Design review of the part built by this model. Coordinates are the model's own, in mm. Face numbers are marked on the shaded views. A direction names the side the tool comes from. Coordinates: 2 decimals unless noted, no trailing zeros. Loops run counter-clockwise (first coordinate to the right, second up) from the corner with the lowest first, then second, coordinate; pieces in that order, holes last. Notation, with made-up numbers: M 71.25,-21 L 104.25,-21 A27 cw 104.25,5 Z; hole C 8.25,79.5 d11. An arc over 180 degrees is marked long. Write item = value, one per line. Start each with the question number.
Autodesk Inventor part; units mm, degrees
ref_plane "YZ Plane" through (0, 0, 0) normal (1, 0, 0) x (0, 1, 0)
ref_plane "XZ Plane" through (0, 0, 0) normal (0, 1, 0) x (-1, 0, 0)
ref_plane "XY Plane" through (0, 0, 0) normal (0, 0, 1) x (1, 0, 0)
sketch "Skizze1" plane through (0, 0, 0) normal (1, 0, 0) x (0, 1, 0)
  line L0 (-12.2718, -10.7427) -> (15.7282, -10.7427)
  line L1 (15.7282, -10.7427) -> (15.7282, -12.7427)
  line L2 (15.7282, -12.7427) -> (-14.2718, -12.7427)
  line L3 (-14.2718, -12.7427) -> (-14.2718, 3.7136)
  line L4 (-14.2718, -12.7427) -> (-6.9903, -12.7427)
  line L5 (-12.2718, -10.7427) -> (-12.2718, 17.2573)
  line L6 (-12.2718, 17.2573) -> (-14.2718, 17.2573)
  line L7 (-14.2718, 17.2573) -> (-14.2718, -12.7427)
  point P0 (0, 0)
  dimension "d0" = 30
  dimension "d1" = 30
  dimension "d2" = 2
  dimension "d3" = 2
extrude "Extrusion1" add sketch "Skizze1" along normal mid plane 30
properties part number "Winkel"
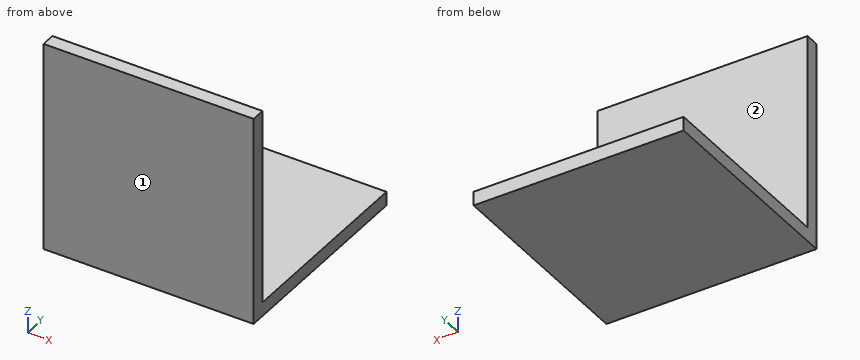
Q1. Add section B-B on x = 3. State the section outline as (y, z) points.
Q2. Add section A-A on y = 7.5. State the section outline as (x, z) points, plus the area to 3 significant figures.
Q3. To check wall thickness, follow line 1 (Y direction, x = 1, z = 8.25); line 2 (Z direction, x = -6, y = -7.5). State the ranges of each line that lie inside material, in increasing order. Write a range as from..to.
Q4. For the marked faces 1 and 2, list the 3-axis set-ups (+Z, -Z, +X, -X, +Y, -Y) from which the entire face can be reached by the end or side of a thin tool; tool diameter is ignored.
Q5. Add section C-C on z = 7. State the section outline as (x, y) points.
Q6. Clearance check with flat-ended pins moving along their axes: P1, Ø4, axis at x = 12, y = -8, coming from the +Z side; P2, Ø4, axis at x = -2.5, z = -2.5, coming from the +Y side. State where each tip first meets the part, or that it passes through.
Values follow:
q1.outline = M -14.27,-12.74 L 15.73,-12.74 L 15.73,-10.74 L -12.27,-10.74 L -12.27,17.26 L -14.27,17.26 Z
q2.outline = M -15,-12.74 L 15,-12.74 L 15,-10.74 L -15,-10.74 Z
q2.area = 60.0 mm2
q3.line_1 = -14.27..-12.27
q3.line_2 = -12.74..-10.74
q4.face_1 = +Z, -Z, +X, -X, -Y
q4.face_2 = +Z, +X, -X, +Y
q5.outline = M -15,-14.27 L 15,-14.27 L 15,-12.27 L -15,-12.27 Z
q6.P1 = -10.74
q6.P2 = -12.27
